from build123d import *

# Parameters (mm, degrees)
SKETCH1_R               = 14.28115
SKETCH1_R_2             = 19.2405
BOSS_EXTRUDE1_DEPTH     = 3.175
F_10_CLEARANCE_HOLE1_D  = 5.1054
F_1_4_CLEARANCE_HOLE1_D = 6.7564
SKETCH6_R               = 2.5527
CUT_EXTRUDE1_DEPTH      = 4.175
FILLET1_R               = 7.62
BOSS_EXTRUDE3_DEPTH     = 3.175
FILLET2_R               = 5.08
F_1_4_CLEARANCE_HOLE2_D = 6.7564


with BuildPart() as part:
    # Sketch1 → Boss-Extrude1 (new body)
    with BuildSketch(Plane(origin=(0, 0, 0), x_dir=(1, 0, 0), z_dir=(0, 1, 0))):
        with BuildLine():
            Line((85.884602434, 50.671947857), (-3.15409287, 44.337954375))
            ThreePointArc((-3.15409287, 44.337954375), (-44.45, 0), (-3.15409287, -44.337954375))
            Line((-3.15409287, -44.337954375), (85.884602434, -50.671947857))
            ThreePointArc((85.884602434, -50.671947857), (140.28928, 0), (85.884602434, 50.671947857))
        make_face()
        with Locations((89.48928, 0)):
            Circle(SKETCH1_R, mode=Mode.SUBTRACT)
        Circle(SKETCH1_R_2, mode=Mode.SUBTRACT)
    extrude(amount=BOSS_EXTRUDE1_DEPTH)

    # #10 Clearance Hole1 (through all)
    with Locations(Plane(origin=(0, 3.175, 0), x_dir=(1, 0, 0), z_dir=(0, 1, 0))):
        with Locations((0, 25.4), (25.4, 0), (0, -25.4), (-25.4, 0)):
            Hole(F_10_CLEARANCE_HOLE1_D / 2)

    # 1/4 Clearance Hole1 (through all)
    with Locations(Plane(origin=(0, 3.175, 0), x_dir=(1, 0, 0), z_dir=(0, 1, 0))):
        with Locations((54.56428, 34.925), (54.56428, -34.925), (114.88928, 25.4), (114.88928, -25.4), (-38.1, 0), (34.925, -34.314713318), (34.925, 34.314713318)):
            Hole(F_1_4_CLEARANCE_HOLE1_D / 2)

    # Sketch6 → Cut-Extrude1 (cut, through all)
    with BuildSketch(Plane(origin=(0, 3.175, 0), x_dir=(1, 0, 0), z_dir=(0, 1, 0))):
        with BuildLine():
            Line((5.08, 18.55775957), (5.08, 25.4))
            ThreePointArc((5.08, 25.4), (0, 30.48), (-5.08, 25.4))
            Line((-5.08, 25.4), (-5.08, 18.55775957))
            ThreePointArc((-5.08, 18.55775957), (0, 19.2405), (5.08, 18.55775957))
        make_face()
        with Locations((0, 25.4)):
            Circle(SKETCH6_R, mode=Mode.SUBTRACT)
        with BuildLine():
            ThreePointArc((5.08, -18.55775957), (0, -19.2405), (-5.08, -18.55775957))
            Line((-5.08, -18.55775957), (-5.08, -25.4))
            ThreePointArc((-5.08, -25.4), (0, -30.48), (5.08, -25.4))
            Line((5.08, -25.4), (5.08, -18.55775957))
        make_face()
        with Locations((0, -25.4)):
            Circle(SKETCH6_R, mode=Mode.SUBTRACT)
    extrude(amount=-CUT_EXTRUDE1_DEPTH, mode=Mode.SUBTRACT)

    # Fillet1
    fillet1_edges = [part.edges().sort_by_distance(p)[0] for p in [
        (-5.08, 1.5875, 18.55775957),
        (5.08, 1.5875, 18.55775957),
        (5.08, 1.5875, -18.55775957),
        (-5.08, 1.5875, -18.55775957),
    ]]
    fillet(fillet1_edges, radius=FILLET1_R)

    # Sketch8 → Boss-Extrude3 (add)
    with BuildSketch(Plane(origin=(0, 3.175, 0), x_dir=(1, 0, 0), z_dir=(0, 1, 0))):
        with BuildLine():
            Line((114.539380559, -44.194258247), (115.971392847, -48.012957682))
            ThreePointArc((115.971392847, -48.012957682), (111.326322318, -58.232112847), (101.107167153, -53.587042318))
            Line((101.107167153, -53.587042318), (99.675154865, -49.768342882))
            ThreePointArc((99.675154865, -49.768342882), (107.326350833, -47.565522221), (114.539380559, -44.194258247))
        make_face()
        with BuildLine():
            Line((99.675154865, 49.768342882), (101.107167153, 53.587042318))
            ThreePointArc((101.107167153, 53.587042318), (111.326322318, 58.232112847), (115.971392847, 48.012957682))
            Line((115.971392847, 48.012957682), (114.539380559, 44.194258247))
            ThreePointArc((114.539380559, 44.194258247), (107.326350833, 47.565522221), (99.675154865, 49.768342882))
        make_face()
        with BuildLine():
            Line((-9.444374405, -43.435081353), (-11.130282191, -47.494435543))
            ThreePointArc((-11.130282191, -47.494435543), (-21.505155543, -51.780437809), (-25.791157809, -41.405564457))
            Line((-25.791157809, -41.405564457), (-24.105250023, -37.346210267))
            ThreePointArc((-24.105250023, -37.346210267), (-17.048839039, -41.050451732), (-9.444374405, -43.435081353))
        make_face()
        with BuildLine():
            Line((-9.444374405, 43.435081353), (-11.130282191, 47.494435543))
            ThreePointArc((-11.130282191, 47.494435543), (-21.505155543, 51.780437809), (-25.791157809, 41.405564457))
            Line((-25.791157809, 41.405564457), (-24.105250023, 37.346210267))
            ThreePointArc((-24.105250023, 37.346210267), (-17.048839039, 41.050451732), (-9.444374405, 43.435081353))
        make_face()
    extrude(amount=-BOSS_EXTRUDE3_DEPTH)

    # Fillet2
    fillet2_edges = [part.edges().sort_by_distance(p)[0] for p in [
        (99.675154865, 1.5875, -49.768342882),
        (114.539380559, 1.5875, -44.194258247),
        (-9.444374405, 1.5875, -43.435081353),
        (-24.105250023, 1.5875, -37.346210267),
        (-24.105250023, 1.5875, 37.346210267),
        (-9.444374405, 1.5875, 43.435081353),
        (114.539380559, 1.5875, 44.194258247),
        (99.675154865, 1.5875, 49.768342882),
    ]]
    fillet(fillet2_edges, radius=FILLET2_R)

    # 1/4 Clearance Hole2 (through all)
    with Locations(Plane(origin=(0, 3.175, 0), x_dir=(1, 0, 0), z_dir=(0, 1, 0))):
        with Locations((108.53928, -50.8), (-18.46072, -44.45), (-18.46072, 44.45), (108.53928, 50.8)):
            Hole(F_1_4_CLEARANCE_HOLE2_D / 2)


solid = part.part
The listing builds one solid part. Answer for the finished solid, in the listing's coordinates (mm). A direction names the side the tool comes from. Give positions to 0.01 mm unless a question says otherwise; leave off trailing zeros. Write each loop counter-clockwise with the first axis right and the second up, starting at its lowest first coordinate (ties: lowest second). Pieces come first, ordered by that corner, then holes. Notation, with made-up numbers: (80.25, -20) - (124.25, -20) arc R32 ccw to (124.25, 6) - close; hole circle Ø2 at (38.5, 70). An arc over 180 degrees is marked (long way). Use a Markdown table: item, result.
1. Section A-A on z = 0 is taken. Count the separate pieces of the cut face and the enclosed holes in it, plus the area to 3 significant figures.
Values follow:
| item | result |
|---|---|
| separate pieces | 6 |
| enclosed holes | 0 |
| area | 320 mm² |
2. Section B-B on x = -38.1 is taken. Write down the section's boundary in (y, z) (3 decimals), plus the area to 3 significant figures.
Values follow:
| item | result |
|---|---|
| outline | (0, -22.895) - (3.175, -22.895) - (3.175, -3.378) - (0, -3.378) - close; (0, 3.378) - (3.175, 3.378) - (3.175, 22.895) - (0, 22.895) - close |
| area | 124 mm² |
3. Find the intervals of material crossed by probe 1 along X at (y, z) = (2.7, 1.5); probe 2 along X at (y, z) = (2.2, -25.4); probe 3 along X at (y, z) = (2.25, -51), in increasing order. Write a range as from..to.
Values follow:
| item | result |
|---|---|
| probe 1 | x = -44.42..-41.13, -35.07..-27.47, -23.33..-19.18, 19.18..23.33, 27.47..75.29, 103.69..140.27 |
| probe 2 | x = -36.48..-5.08, 5.08..111.51, 118.27..133.48 |
| probe 3 | x = -22.94..-13.98, 98.83..105.17, 111.91..116.47 |
4. Section D-D on x = 83.5 is taken. Write down the section's boundary in (y, z) (3 decimals), plus the area to 3 significant figures.
Values follow:
| item | result |
|---|---|
| outline | (0, -50.502) - (3.175, -50.502) - (3.175, -12.965) - (0, -12.965) - close; (0, 12.965) - (3.175, 12.965) - (3.175, 50.502) - (0, 50.502) - close |
| area | 238 mm² |
5. Each of these flat-tipped pins is pushed along its axis until it touches: P1, Ø1.9, axis at y = 2, z = 24.5, coming from the -X side; P2, Ø0.5, axis at y = 1.5, z = -25, coming from the +X side; P3, Ø1.9, axis at y = 1.5, z = -24, coming from the -X side. Where does it stop, or does it pass through?
Values follow:
| item | result |
|---|---|
| P1 | stops at x = -37.7 |
| P2 | stops at x = 133.85 |
| P3 | stops at x = -38.01 |
6. For a pull along X with two mould halves and no side action, classify faces 4 (the cylindrical face through (111.49, 1.61, 58.17)), 5 (the cylindrical face through (33.366, 1.565, 37.312)), 6 (the cylindrical face through (-44.446, 1.565, -0.567)) as released by +X, released by -X, zero draft, split by the parting line, or undercut.
Values follow:
| item | result |
|---|---|
| face 4 | split by the parting line |
| face 5 | undercut |
| face 6 | released by -X |
7. A tool of negligible diameter and unlimited length cuts with its end or side. For faces 1 (the flat face through (40.74, 1.57, 47.46)), 2 (the flat face through (41.99, 1.57, -47.55)), 3 (the cylindrical face through (-19.24, 1.57, -0.29)), from which of +Z, -Z, +X, -X, +Y, -Y can it reach the whole face along a straight path? Write none if from no direction.
Values follow:
| item | result |
|---|---|
| face 1 | +Z, +Y, -Y |
| face 2 | -Z, +Y, -Y |
| face 3 | +Y, -Y |
